from build123d import *

# Parameters (mm, degrees)
BOSS_EXTRUDE1_DEPTH = 4
BOSS_EXTRUDE2_DEPTH = 37.5
SKETCH7_R           = 5
CUT_EXTRUDE1_DEPTH  = 30


with BuildPart() as part:
    # Sketch1 → Boss-Extrude1 (new body)
    with BuildSketch(Plane.XY):
        with BuildLine():
            Line((0, 0), (70, 0))
            Line((70, 0), (70, 100))
            Line((70, 100), (40, 100))
            Line((40, 100), (18.812777554, 54.710910751))
            Line((18.812777554, 54.710910751), (18.812777554, 39.710910751))
            ThreePointArc((18.812777554, 39.710910751), (1.181989874, 23.75170918), (0, 0))
        make_face()
    extrude(amount=BOSS_EXTRUDE1_DEPTH)

    # Sketch5 → Boss-Extrude2 (add)
    with BuildSketch(Plane(origin=(18.8, 0, 0), x_dir=(0, 0, -1), z_dir=(1, 0, 0))):
        with BuildLine():
            Line((-4, 54.710910751), (-4, 39.710910751))
            ThreePointArc((-4, 39.710910751), (-11.5, 47.210910751), (-4, 54.710910751))
        make_face()
    extrude(amount=BOSS_EXTRUDE2_DEPTH)

    # Sketch7 → Cut-Extrude1 (cut)
    with BuildSketch(Plane(origin=(18.8, 0, 0), x_dir=(0, 0, -1), z_dir=(1, 0, 0))):
        with Locations(Location((-5.690630422, 47.210910751, 0), (0, 0, 289.762746065))):
            Circle(SKETCH7_R)
    extrude(amount=CUT_EXTRUDE1_DEPTH, mode=Mode.SUBTRACT)


solid = part.part
Verification items for the finished model (mm, model axes). A direction names the side the tool comes from. Coordinates: 2 decimals unless noted, no trailing zeros. Order: outer loops, then holes, each group sorted by start corner. A loop starts at its lowest first (then second) coordinate and runs counter-clockwise, first axis right, second up.
1. Sectioned sample at A-A, the plane x = 46. Record the cut outline in (y, z), and give its area (3 significant figures).
Results found:
outline: (0, 0) - (100, 0) - (100, 4) - (54.71, 4) arc R7.5 ccw to (39.71, 4) - (0, 4) - close; hole circle Ø10 at (47.21, 5.69)
area: 410 mm2
2. Sectioned sample at C-C, the plane y = 46.5. Record the cut outline in (x, z), and give its area (3 significant figures).
Results found:
outline: (18.8, 10.64) - (48.8, 10.64) - (48.8, 0.74) - (18.81, 0.74) - (18.81, 0) - (70, 0) - (70, 4) - (56.3, 4) - (56.3, 11.47) - (18.8, 11.47) - close
area: 188 mm2
3. Sectioned sample at D-D, the plane x = 26.5. Record the cut outline in (y, z).
Results found:
outline: (0, 0) - (71.14, 0) - (71.14, 4) - (54.71, 4) arc R7.5 ccw to (39.71, 4) - (0, 4) - close; hole circle Ø10 at (47.21, 5.69)
4. Go/stop test with flat-tipped pins: pin 1 Ø5 at (x, z) = (36.5, 2.5) entering from +Y; pin 2 Ø1.2 at (y, z) = (49.5, 2.5) entering from -X; pin 3 Ø5 at (y, z) = (13.5, 7) entering from +X; pin 4 Ø1 at (x, z) = (29.5, 8.5) entering from -Y. Record where each tip stops, or that it passes through.
Results found:
pin 1: stops at y = 97.86
pin 2: stops at x = 48.8
pin 3: passes through
pin 4: stops at y = 40.87
5. Release check for a two-part mould opening along Y. For faces 3 (the face through (35, 0, 2)), 4 (the face through (48.8, 47, 6)), 5 (the face through (70, 49, 2)) record: +Y half, -Y half, draft (parallel to the pull), parting line (faces both ways), or undercut.
Results found:
face 3: -Y half
face 4: undercut
face 5: draft
6. Scan lines: line 1 (Z direction, x = 56.5, y = 50.5); line 2 (Y direction, x = 38, z = 2.5); line 3 (Y direction, x = 32.5, z = 1.25). Record each from-to range of solid material in increasing order.
Results found:
line 1: z = 0 to 4
line 2: y = 0 to 43.36, 51.06 to 95.72
line 3: y = 0 to 44.91, 49.51 to 83.97
7. Sectioned sample at B-B, the plane z = 5. Record the cut outline in (x, y), and give its area (3 significant figures).
Results found:
outline: (18.8, 39.78) - (56.3, 39.78) - (56.3, 54.64) - (18.8, 54.64) - (18.8, 52.16) - (48.8, 52.16) - (48.8, 42.26) - (18.8, 42.26) - close
area: 260 mm2
8. Set-up check for faces 1 (the face through (33.59, 42.217, 5.931)), 2 (the face through (56.3, 47, 7)): record each of +Z, -Z, +X, -X, +Y, -Y from which the full face is reachable in a straight line by a thin tool's end or side.
Results found:
face 1: -X
face 2: +Z, +X, +Y, -Y
